from build123d import *

# Parameters (mm, degrees)
SKETCH1_R           = 16
SKETCH1_R_2         = 2
BOSS_EXTRUDE1_DEPTH = 8
SKETCH4_R           = 16
SKETCH4_R_2         = 11
BOSS_EXTRUDE3_DEPTH = 5
SKETCH5_R           = 1.5
CUT_EXTRUDE2_DEPTH  = 9
SKETCH6_R           = 3.175
CUT_EXTRUDE3_DEPTH  = 6
SKETCH7_OUTSIDE_W   = 86.584
SKETCH7_OUTSIDE_H   = 82.792
SKETCH7_OUTSIDE_R   = 19.075
CUT_EXTRUDE4_DEPTH  = 3


with BuildPart() as part:
    # Sketch1 → Boss-Extrude1 (new body)
    with BuildSketch(Plane(origin=(0, 0, 0), x_dir=(1, 0, 0), z_dir=(0, 1, 0))):
        with BuildLine():
            Line((30.645825623, -11.919872981), (26.994897428, -9.812008605))
            ThreePointArc((26.994897428, -9.812008605), (24.953655976, -7.574039819), (24.57908119, -4.568234655))
            ThreePointArc((24.57908119, -4.568234655), (21.650635095, 12.5), (8.333333333, 23.57022604))
            ThreePointArc((8.333333333, 23.57022604), (5.917517095, 25.397519902), (5, 28.284271247))
            Line((5, 28.284271247), (5, 32.5))
            ThreePointArc((5, 32.5), (0, 37.5), (-5, 32.5))
            Line((-5, 32.5), (-5, 28.284271247))
            ThreePointArc((-5, 28.284271247), (-5.917517095, 25.397519902), (-8.333333333, 23.57022604))
            ThreePointArc((-8.333333333, 23.57022604), (-21.650635095, 12.5), (-24.57908119, -4.568234655))
            ThreePointArc((-24.57908119, -4.568234655), (-24.953655976, -7.574039819), (-26.994897428, -9.812008605))
            Line((-26.994897428, -9.812008605), (-30.645825623, -11.919872981))
            ThreePointArc((-30.645825623, -11.919872981), (-32.475952642, -18.75), (-25.645825623, -20.580127019))
            Line((-25.645825623, -20.580127019), (-21.994897428, -18.472262643))
            ThreePointArc((-21.994897428, -18.472262643), (-19.03613888, -17.823480083), (-16.245747857, -19.001991385))
            ThreePointArc((-16.245747857, -19.001991385), (0, -25), (16.245747857, -19.001991385))
            ThreePointArc((16.245747857, -19.001991385), (19.03613888, -17.823480083), (21.994897428, -18.472262643))
            Line((21.994897428, -18.472262643), (25.645825623, -20.580127019))
            ThreePointArc((25.645825623, -20.580127019), (32.475952642, -18.75), (30.645825623, -11.919872981))
        make_face()
        Circle(SKETCH1_R, mode=Mode.SUBTRACT)
        with Locations((0, 32.5)):
            Circle(SKETCH1_R_2, mode=Mode.SUBTRACT)
        with Locations((-28.145825623, -16.25)):
            Circle(SKETCH1_R_2, mode=Mode.SUBTRACT)
        with Locations((28.145825623, -16.25)):
            Circle(SKETCH1_R_2, mode=Mode.SUBTRACT)
    extrude(amount=BOSS_EXTRUDE1_DEPTH)

    # Sketch4 → Boss-Extrude3 (add)
    with BuildSketch(Plane(origin=(0, 8, 0), x_dir=(1, 0, 0), z_dir=(0, 1, 0))):
        Circle(SKETCH4_R)
        Circle(SKETCH4_R_2, mode=Mode.SUBTRACT)
    extrude(amount=-BOSS_EXTRUDE3_DEPTH)

    # Sketch5 → Cut-Extrude2 (cut, through all)
    with BuildSketch(Plane(origin=(0, 8, 0), x_dir=(1, 0, 0), z_dir=(0, 1, 0))):
        with Locations((0, -14)):
            Circle(SKETCH5_R)
        with Locations((-12.124355653, 7)):
            Circle(SKETCH5_R)
        with Locations((12.124355653, 7)):
            Circle(SKETCH5_R)
    extrude(amount=-CUT_EXTRUDE2_DEPTH, mode=Mode.SUBTRACT)

    # Sketch6 → Cut-Extrude3 (cut)
    with BuildSketch(Plane.XZ):
        with Locations((0, 14)):
            Circle(SKETCH6_R)
        with Locations((-12.124355653, -7)):
            Circle(SKETCH6_R)
        with Locations((12.124355653, -7)):
            Circle(SKETCH6_R)
    extrude(amount=-CUT_EXTRUDE3_DEPTH, mode=Mode.SUBTRACT)

    # Sketch7 outside → Cut-Extrude4 (cut)
    with BuildSketch(Plane(origin=(0, 8, 0), x_dir=(1, 0, 0), z_dir=(0, 1, 0))):
        with Locations((0, 6.25)):
            Rectangle(SKETCH7_OUTSIDE_W, SKETCH7_OUTSIDE_H)
        Circle(SKETCH7_OUTSIDE_R, mode=Mode.SUBTRACT)
    extrude(amount=-CUT_EXTRUDE4_DEPTH, mode=Mode.SUBTRACT)


solid = part.part
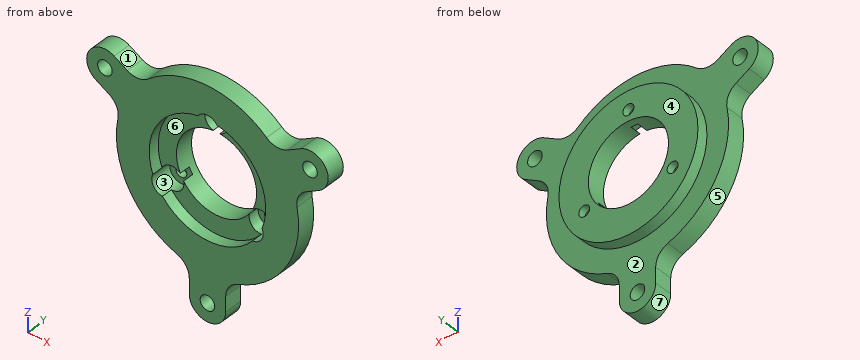
Work out the finished part from the listing and answer in its coordinate system (mm). Face numbers are marked on the shaded views. A direction names the side the tool comes from. Coordinates: 2 decimals unless noted, no trailing zeros. Loops run counter-clockwise (first coordinate to the right, second up) from the corner with the lowest first, then second, coordinate; pieces in that order, holes last. Notation, with made-up numbers: M 3.5,5.5 L 26.5,5.5 A14 ccw 26.5,17.5 Z; hole C 73.25,16.25 d1. An arc over 180 degrees is marked long. Answer in a Markdown table with one row per item. Add a question column.
1. Find section D-D, the plane x = 18. Write down the section's boundary in (y, z), then the cut area to 3 significant figures.
2. The mould has two halves that part along X. Classify the marked faces 4, 5, 6 and 7: pulls with the +X half, pulls with the -X half, needs draft (parallel to the pull), parting line crosses it, or undercut.
3. Consider L1, parallel to Z at x = 0, y = 7.3 (3 decimals); L2, parallel to X at y = 2.65, z = 16.25; L3, parallel to X at y = 2.55, z = -32.5. Determine where each line is inside the solid, lowest interval first.
4. Find section B-B, the plane z = 0. Write down the section's boundary in (x, y) (3 decimals).
5. A tool of negligible diameter and unlimited length cuts with its end or side. For the marked faces 1, 2 and 3, from which of +Z, -Z, +X, -X, +Y, -Y can it reach the whole face along a straight path? Write none if from no direction.
6. Find section A-A, the plane x = 0. Write down the section's boundary in (y, z) (3 decimals).
7. Find section C-C, the plane y = 1.25. Write down the section's boundary in (x, z) (3 decimals).
8. Flat-ended cylindrical pins translate along their axes: P1, Ø7.5, axis at x = 11.5, z = 9, coming from the -Y side; P2, Ø2, axis at x = 18, y = 1.5, coming from the -Z side; P3, Ø7.5, axis at x = -9.5, z = 2.5, coming from the -Y side; P4, Ø1, axis at x = 23, y = 5, coming from the -Z side. Find the tip coordinate at first contact, or state that the pin passes through.
Reported:
| question | item | result |
|---|---|---|
| 1 | outline | M 0,-17.35 L 5,-17.35 L 5,-6.31 L 8,-6.31 L 8,6.31 L 5,6.31 L 5,18.03 L 0,18.03 Z |
| 1 | area | 215 mm^2 |
| 2 | face 4 | needs draft |
| 2 | face 5 | pulls with the -X half |
| 2 | face 6 | undercut |
| 2 | face 7 | parting line crosses it |
| 3 | L1 | z = -19.075 to -11, 11 to 12.5, 15.5 to 19.075 |
| 3 | L2 | x = -33.15 to -30.15, -26.15 to -2.24, 2.24 to 26.15, 30.15 to 33.15 |
| 3 | L3 | x = -5 to -2, 2 to 5 |
| 4 | outline | M -25,0 L -16,0 L -16,3 L -11,3 L -11,8 L -19.075,8 L -19.075,5 L -25,5 Z; M 11,3 L 16,3 L 16,0 L 25,0 L 25,5 L 19.075,5 L 19.075,8 L 11,8 Z |
| 5 | face 1 | +Z, +Y, -Y |
| 5 | face 2 | +Y |
| 5 | face 3 | -Y |
| 6 | outline | M 0,-37.5 L 5,-37.5 L 5,-34.5 L 0,-34.5 Z; M 0,-30.5 L 5,-30.5 L 5,-19.075 L 8,-19.075 L 8,-11 L 3,-11 L 3,-16 L 0,-16 Z; M 0,17.175 L 6,17.175 L 6,15.5 L 8,15.5 L 8,19.075 L 5,19.075 L 5,25 L 0,25 Z; M 6,11 L 8,11 L 8,12.5 L 6,12.5 Z |
| 7 | outline | M -30.646,11.92 L -26.995,9.812 A5 cw -24.579,4.568 A25 ccw -8.333,-23.57 A5 cw -5,-28.284 L -5,-32.5 A5 ccw 5,-32.5 L 5,-28.284 A5 cw 8.333,-23.57 A25 ccw 24.579,4.568 A5 cw 26.995,9.812 L 30.646,11.92 A5 ccw 25.646,20.58 L 21.995,18.472 A5 cw 16.246,19.002 A25 ccw -16.246,19.002 A5 cw -21.995,18.472 L -25.646,20.58 A5 ccw Z; hole C -28.146,16.25 d4; hole M -14.982,-5.616 A3.175 ccw -12.355,-10.167 A16 ccw 12.355,-10.167 A3.175 ccw 14.982,-5.616 A16 ccw 2.627,15.783 A3.175 ccw -2.627,15.783 A16 ccw Z; hole C 0,-32.5 d4; hole C 28.146,16.25 d4 |
| 8 | P1 | stops at y = 0 |
| 8 | P2 | stops at z = -18.33 |
| 8 | P3 | stops at y = 3 |
| 8 | P4 | stops at z = -10.9 |
